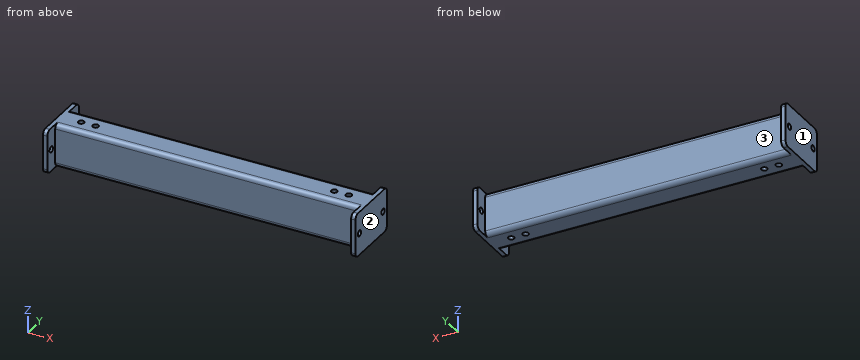
from build123d import *

# Parameters (mm, degrees)
DODANIE_WYCI_GNI_CIE2_DEPTH = 420
SZKIC4_R                    = 4.1
DODANIE_WYCI_GNI_CIE3_DEPTH = 6
DODANIE_WYCI_GNI_CIE4_REACH = 434.06
SZKIC5_R                    = 8.1
SZKIC5_R_2                  = 4.1
SZKIC6_R                    = 4.1
WYTNIJ_WYCI_GNI_CIE1_DEPTH  = 433.060180993


with BuildPart() as part:
    # Szkic3 → Dodanie-wyci_gni_cie2 (new body)
    with BuildSketch(Plane(origin=(0, 0, 0), x_dir=(0, 0, -1), z_dir=(1, 0, 0))):
        with BuildLine():
            Line((-23.6, -20), (23.6, -20))
            ThreePointArc((23.6, -20), (28.1254834, -18.1254834), (30, -13.6))
            Line((30, -13.6), (30, 13.6))
            ThreePointArc((30, 13.6), (28.1254834, 18.1254834), (23.6, 20))
            Line((23.6, 20), (-23.6, 20))
            ThreePointArc((-23.6, 20), (-28.1254834, 18.1254834), (-30, 13.6))
            Line((-30, 13.6), (-30, -13.6))
            ThreePointArc((-30, -13.6), (-28.1254834, -18.1254834), (-23.6, -20))
        make_face()
        with BuildLine():
            Line((-17.6, 14), (17.6, 14))
            ThreePointArc((17.6, 14), (22.1254834, 12.1254834), (24, 7.6))
            Line((24, 7.6), (24, -7.6))
            ThreePointArc((24, -7.6), (22.1254834, -12.1254834), (17.6, -14))
            Line((17.6, -14), (-17.6, -14))
            ThreePointArc((-17.6, -14), (-22.1254834, -12.1254834), (-24, -7.6))
            Line((-24, -7.6), (-24, 7.6))
            ThreePointArc((-24, 7.6), (-22.1254834, 12.1254834), (-17.6, 14))
        make_face(mode=Mode.SUBTRACT)
    extrude(amount=DODANIE_WYCI_GNI_CIE2_DEPTH)

    # Szkic4 → Dodanie-wyci_gni_cie3 (add)
    with BuildSketch(Plane(origin=(420, 0, 0), x_dir=(0, 0, -1), z_dir=(1, 0, 0))):
        with BuildLine():
            Line((-23.6, -40), (23.6, -40))
            ThreePointArc((23.6, -40), (28.1254834, -38.1254834), (30, -33.6))
            Line((30, -33.6), (30, 33.6))
            ThreePointArc((30, 33.6), (28.1254834, 38.1254834), (23.6, 40))
            Line((23.6, 40), (-23.6, 40))
            ThreePointArc((-23.6, 40), (-28.1254834, 38.1254834), (-30, 33.6))
            Line((-30, 33.6), (-30, -33.6))
            ThreePointArc((-30, -33.6), (-28.1254834, -38.1254834), (-23.6, -40))
        make_face()
        with Locations((0, 30)):
            Circle(SZKIC4_R, mode=Mode.SUBTRACT)
        with Locations(Location((0, -30, 0), (0, 0, 180))):
            Circle(SZKIC4_R, mode=Mode.SUBTRACT)
    dodanie_wyci_gni_cie3 = extrude(amount=DODANIE_WYCI_GNI_CIE3_DEPTH)

    # Szkic5 → Dodanie-wyci_gni_cie4 (add, up to next)
    with BuildSketch(Plane.XY.offset(30), mode=Mode.PRIVATE) as dodanie_wyci_gni_cie4_sk1:
        with Locations(Location((25, 0, 0), (0, 0, 69.763291811))):
            Circle(SZKIC5_R)
        with Locations((25, 0)):
            Circle(SZKIC5_R_2, mode=Mode.SUBTRACT)
    dodanie_wyci_gni_cie4_tool1 = extrude(dodanie_wyci_gni_cie4_sk1.sketch, amount=-DODANIE_WYCI_GNI_CIE4_REACH, mode=Mode.PRIVATE) - part.part
    # Szkic5 → Dodanie-wyci_gni_cie4 (add, up to next)
    with BuildSketch(Plane.XY.offset(30), mode=Mode.PRIVATE) as dodanie_wyci_gni_cie4_sk2:
        with Locations(Location((45, 0, 0), (0, 0, 69.763291811))):
            Circle(SZKIC5_R)
        with Locations((45, 0)):
            Circle(SZKIC5_R_2, mode=Mode.SUBTRACT)
    dodanie_wyci_gni_cie4_tool2 = extrude(dodanie_wyci_gni_cie4_sk2.sketch, amount=-DODANIE_WYCI_GNI_CIE4_REACH, mode=Mode.PRIVATE) - part.part
    dodanie_wyci_gni_cie4_1 = dodanie_wyci_gni_cie4_tool1.solids().sort_by_distance((22.277461, -7.38504, 30))[0]
    add(dodanie_wyci_gni_cie4_1)
    dodanie_wyci_gni_cie4_2 = dodanie_wyci_gni_cie4_tool2.solids().sort_by_distance((42.277461, -7.38504, 30))[0]
    add(dodanie_wyci_gni_cie4_2)
    dodanie_wyci_gni_cie4 = dodanie_wyci_gni_cie4_1 + dodanie_wyci_gni_cie4_2  # Dodanie-wyci_gni_cie4 as one shape, for the pattern or mirror that repeats it

    # Szkic6 → Wytnij-wyci_gni_cie1 (cut, through all)
    with BuildSketch(Plane.XY.offset(30)):
        with Locations((25, 0)):
            Circle(SZKIC6_R)
        with Locations((45, 0)):
            Circle(SZKIC6_R)
    wytnij_wyci_gni_cie1 = extrude(amount=-WYTNIJ_WYCI_GNI_CIE1_DEPTH, mode=Mode.SUBTRACT)

    # Lustro3: Dodanie-wyci_gni_cie4, Wytnij-wyci_gni_cie1 across plane
    add(dodanie_wyci_gni_cie4.mirror(Plane(origin=(210, 0, 0), x_dir=(0, 0, 1), z_dir=(1, 0, 0))))
    add(wytnij_wyci_gni_cie1.mirror(Plane(origin=(210, 0, 0), x_dir=(0, 0, 1), z_dir=(1, 0, 0))), mode=Mode.SUBTRACT)

    # Lustro4: Dodanie-wyci_gni_cie3 across plane
    add(dodanie_wyci_gni_cie3.mirror(Plane(origin=(210, 0, 0), x_dir=(0, 0, 1), z_dir=(1, 0, 0))))


solid = part.part
Verification items for the finished model (mm, model axes). Face numbers are marked on the shaded views. Give positions to 0.01 mm unless a question says otherwise; leave off trailing zeros. Write each loop counter-clockwise with the first axis right and the second up, starting at its lowest first coordinate (ties: lowest second). Pieces come first, ordered by that corner, then holes. Notation, with made-up numbers: (51, 27) - (76, 27) arc R25 cw to (76, 50) - close; hole circle Ø10 at (25.5, 81.25). An arc over 180 degrees is marked (long way). Answer as CSV lines item,"result". Start each with the question number.
1. Sectioned sample at A-A (y = -30). Record the boundary of the cut face in (x, z), then the cut area to 3 significant figures.
2. Depth check by flat-ended pin: pin 1 (13 mm diameter, centred on y = -27.5, z = -2.5, fed in from +X); pin 2 (10 mm diameter, centred on x = 44, z = -8.5, fed in from +Y); pin 3 (10.5 mm diameter, centred on x = 191, z = 4.5, fed in from -Y); pin 4 (3 mm diameter, centred on x = 259, y = -18, fed in from +Z). Enter the tip coordinate at first touch or a pass-through.
3. Thickness scan on line 1 (Y direction, x = 45, z = 4); line 2 (X direction, y = -27, z = 3); line 3 (Y direction, x = 123, z = 9). Record the ranges inside material, lowest first.
4. Sectioned sample at B-B (x = 361). Record the boundary of the cut face in (y, z), then the cut area to 3 significant figures.
5. Draft check along X on the marked faces 1, 2 and 3. Enter one of: pulls with the +X half, pulls with the -X half, needs draft (parallel to the pull), parting line crosses it, or undercut.
Derived:
1,outline,"(-6, -30) - (0, -30) - (0, -4.1) - (-6, -4.1) - close; (-6, 4.1) - (0, 4.1) - (0, 30) - (-6, 30) - close; (420, -30) - (426, -30) - (426, -4.1) - (420, -4.1) - close; (420, 4.1) - (426, 4.1) - (426, 30) - (420, 30) - close"
1,area,"622 mm²"
2,pin 1,"x = 426"
2,pin 2,"y = 20"
2,pin 3,"y = -20"
2,pin 4,"z = 29.31"
3,line 1,"-20 to -14, -8.1 to -4.1, 4.1 to 8.1, 14 to 20"
3,line 2,"-6 to 0, 420 to 426"
3,line 3,"-20 to -14, 14 to 20"
4,outline,"(-20, -23.6) arc R6.4 ccw to (-13.6, -30) - (13.6, -30) arc R6.4 ccw to (20, -23.6) - (20, 23.6) arc R6.4 ccw to (13.6, 30) - (-13.6, 30) arc R6.4 ccw to (-20, 23.6) - close; hole (-14, -17.6) arc R6.4 ccw to (-7.6, -24) - (7.6, -24) arc R6.4 ccw to (14, -17.6) - (14, 17.6) arc R6.4 ccw to (7.6, 24) - (-7.6, 24) arc R6.4 ccw to (-14, 17.6) - close"
4,area,"1,060 mm²"
5,face 1,"pulls with the -X half"
5,face 2,"pulls with the +X half"
5,face 3,"undercut"
